from build123d import *

# Parameters (mm, degrees)
F0_W     = 38.1
F0_H     = 13.271
F1_DEPTH = 15.24
F3_DEPTH = 8
F0_H_2   = 5.271
F4_DEPTH = 15.24
F5_R     = 4.5
F6_DEPTH = 16.002


with BuildPart() as f1:
    # F0 (on Top) → F1 (new body)
    with BuildSketch(Plane.XY):
        with Locations((0, 2.6355)):
            Rectangle(F0_W, F0_H)
    extrude(amount=F1_DEPTH)

    # F2 (on face) → F3 (cut)
    with BuildSketch(Plane.XZ.offset(4)):
        with BuildLine():
            Line((8.45, 0), (15.45, 0))
            ThreePointArc((15.45, 0), (3.95, 11.5), (-7.55, 0))
            Line((-7.55, 0), (-0.55, 0))
            ThreePointArc((-0.55, 0), (3.95, 4.5), (8.45, 0))
        make_face()
        with BuildLine():
            Line((-0.55, 0), (8.45, 0))
            ThreePointArc((8.45, 0), (3.95, 4.5), (-0.55, 0))
        make_face()
    extrude(amount=-F3_DEPTH, mode=Mode.SUBTRACT)

    # F0 (on Top) → F4 (join)
    with BuildSketch(Plane.XY):
        with Locations((0, -6.6355)):
            Rectangle(F0_W, F0_H_2)
    extrude(amount=F4_DEPTH)

    # F5 (on face) → F6 (cut)
    with BuildSketch(Plane.XZ.offset(9.271)):
        with Locations((3.95, 0)):
            Circle(F5_R)
    extrude(amount=-F6_DEPTH, mode=Mode.SUBTRACT)


solid = f1.part
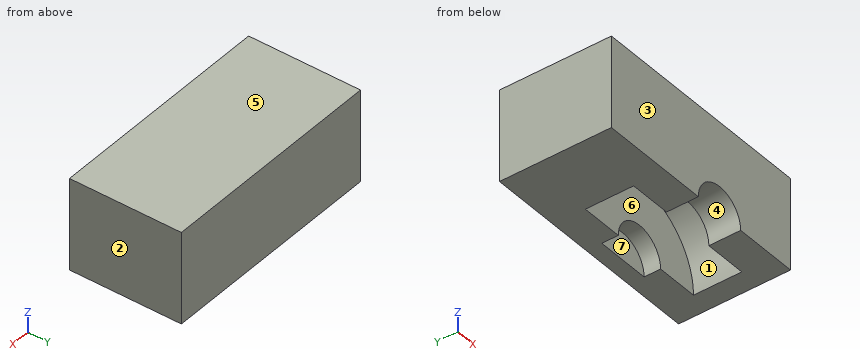
Source: CAD feature listing. Evaluate the final solid. Frame: model axes, mm. Face numbers are marked on the shaded views. A direction names the side the tool comes from. Round coordinates to 2 decimals unless told otherwise and drop trailing zeros. Loops run counter-clockwise (first coordinate to the right, second up) from the corner with the lowest first, then second, coordinate; pieces in that order, holes last. Notation, with made-up numbers: M -14,-29 L -9,-29 A19 ccw -9,-6 Z; hole C 26,8.5 d6. An arc over 180 degrees is marked long. Answer as CSV lines item,"result".
Q1. Cut plane D-D (z = 1.75). Return the cut outline in (x, y).
Verdict:
outline,"M -19.05,-9.27 L -0.2,-9.27 L -0.2,-4 L -7.42,-4 L -7.42,4 L -0.2,4 L -0.2,6.73 L 8.1,6.73 L 8.1,4 L 15.32,4 L 15.32,-4 L 8.1,-4 L 8.1,-9.27 L 19.05,-9.27 L 19.05,9.27 L -19.05,9.27 Z"
Q2. Cut plane A-A (z = 8). Return the cut outline in (x, y).
Verdict:
outline,"M -19.05,-9.27 L 19.05,-9.27 L 19.05,9.27 L -19.05,9.27 Z; hole M -4.31,-4 L 12.21,-4 L 12.21,4 L -4.31,4 Z"
Q3. Contact query for flat-ended pins moving along their axis: pin 1 (5 mm diameter, centred on x = 5, z = 1.5, fed in from -Y); pin 2 (1.5 mm diameter, centred on x = 11.5, y = 2.5, fed in from -Z). Output: stop coordinate, or through.
Verdict:
pin 1,"stops at y = 6.73"
pin 2,"stops at z = 7.96"
Q4. Reachability of the marked faces 5, 6 and 7 from +Z, -Z, +X, -X, +Y, -Y: full face, straight path, thin tool, end or side. Return the list, or none.
Verdict:
face 5,"+Z, +X, -X, +Y, -Y"
face 6,"-Z"
face 7,"-Z, -Y"
Q5. Pull-direction query (X, two-part tool) for the marked faces 1, 2, 3 and 4; classes: +X half, -X half, draft (parallel to the pull), parting line (faces both ways), or undercut.
Verdict:
face 1,"undercut"
face 2,"+X half"
face 3,"draft"
face 4,"undercut"
Q6. Cut plane C-C (y = 0.75). Return the cut outline in (x, z), plus the area to 3 significant figures.
Verdict:
outline,"M -19.05,0 L -7.55,0 A11.5 cw 15.45,0 L 19.05,0 L 19.05,15.24 L -19.05,15.24 Z"
area,"373 mm^2"
Q7. Line query: line 1 along Y through (x, z) = (13, 1.5); line 2 along Y through (x, z) = (7, 0.75); line 3 along Z through (x, y) = (6, 6.5). Output: solid intervals per line, ascending.
Verdict:
line 1,"y = -9.27 to -4, 4 to 9.27"
line 2,"y = 6.73 to 9.27"
line 3,"z = 4.01 to 15.24"
Q8. Cut plane B-B (x = 3.95). Return the cut outline in (y, z), plus the area to 3 significant figures.
Verdict:
outline,"M -9.27,4.5 L -4,4.5 L -4,11.5 L 4,11.5 L 4,4.5 L 6.73,4.5 L 6.73,0 L 9.27,0 L 9.27,15.24 L -9.27,15.24 Z"
area,"155 mm^2"
